Design review of the part built by this model. Coordinates are the model's own, in mm. A direction names the side the tool comes from. Round coordinates to 2 decimals unless told otherwise and drop trailing zeros. Order: outer loops, then holes, each group sorted by start corner. A loop starts at its lowest first (then second) coordinate and runs counter-clockwise, first axis right, second up. Notation, with made-up numbers: (22.5, -34) - (55.5, -34) arc R14 ccw to (55.5, -11) - close; hole circle Ø1 at (78.25, 83). An arc over 180 degrees is marked (long way). Use CSV: the item, a comma, the result in double quotes. Start each with the question number.
from build123d import *

# Parameters (mm, degrees)
BOSS_EXTRUDE3_DEPTH                    = 210
FILLET1_R                              = 2.5
FILLET2_R                              = 12.5
CHAMFER1_SIZE                          = 1
M10_TAPPED_HOLE1_D                     = 8.5
M10_TAPPED_HOLE1_DEPTH                 = 27.5
M10_TAPPED_HOLE1_CSINK_D               = 10.05
M10_TAPPED_HOLE1_CSINK_ANGLE           = 100
M10_TAPPED_HOLE1_TIP                   = 2.553657631
M10_TAPPED_HOLE1_ON_FACE_2_D           = 8.5
M10_TAPPED_HOLE1_ON_FACE_2_DEPTH       = 27.5
M10_TAPPED_HOLE1_ON_FACE_2_CSINK_D     = 10.05
M10_TAPPED_HOLE1_ON_FACE_2_CSINK_ANGLE = 100
M10_TAPPED_HOLE1_ON_FACE_2_TIP         = 2.553657631
CUT_EXTRUDE1_DEPTH                     = 9


with BuildPart() as part:
    # Sketch1 → Boss-Extrude3 (new, symmetric)
    with BuildSketch(Plane(origin=(0, 0, 0), x_dir=(0, 0, -1), z_dir=(1, 0, 0))):
        Polygon((23.094010768, -40), (46.188021535, 0), (23.094010768, 40), (-23.094010768, 40), (-46.188021535, 0), (-23.094010768, -40), align=None)
    extrude(amount=BOSS_EXTRUDE3_DEPTH, both=True)

    # Sketch3 → Revolve1 (revolve)
    with BuildSketch(Plane.XY, mode=Mode.PRIVATE) as revolve1_sk:
        Polygon((-210, 35), (-240, 35), (-240, 32.5), (-265, 32.5), (-265, 0), (-210, 0), align=None)
        Polygon((210, 35), (240, 35), (240, 32.5), (320, 32.5), (320, 30), (420, 30), (420, 0), (210, 0), align=None)
    revolve(revolve1_sk.sketch.rotate(Axis((-265, 0, 0), (1, 0, 0)), 90), axis=Axis((-265, 0, 0), (1, 0, 0)))

    # Fillet1
    fillet1_edges = [part.edges().sort_by_distance(p)[0] for p in [
        (-210, 0, -35),
        (-240, 0, -32.5),
        (210, 0, -35),
        (240, 0, -32.5),
    ]]
    fillet(fillet1_edges, radius=FILLET1_R - 0.0001)  # a hair under: the kernel refuses the full size

    # Fillet2
    fillet2_edges = [part.edges().sort_by_distance(p)[0] for p in [
        (0, -40, 23.094010768),
        (0, 0, 46.188021535),
        (0, 40, 23.094010768),
        (0, 40, -23.094010768),
        (0, 0, -46.188021535),
        (0, -40, -23.094010768),
    ]]
    fillet(fillet2_edges, radius=FILLET2_R)

    # Chamfer1
    chamfer1_edges = [part.edges().sort_by_distance(p)[0] for p in [
        (-265, 0, -32.5),
        (320, 0, -32.5),
        (420, 0, -30),
    ]]
    chamfer(chamfer1_edges, length=CHAMFER1_SIZE)

    # M10 Tapped Hole1
    with Locations(Plane(origin=(-265, 0, 0), x_dir=(0, 0, -1), z_dir=(-1, 0, 0))):
        with Locations((0, 0)):
            CounterSinkHole(M10_TAPPED_HOLE1_D / 2, M10_TAPPED_HOLE1_CSINK_D / 2, depth=M10_TAPPED_HOLE1_DEPTH, counter_sink_angle=M10_TAPPED_HOLE1_CSINK_ANGLE)
            with Locations((0, 0, -(M10_TAPPED_HOLE1_DEPTH + M10_TAPPED_HOLE1_TIP / 2))):  # 118° drill point
                Cone(0, M10_TAPPED_HOLE1_D / 2, M10_TAPPED_HOLE1_TIP, mode=Mode.SUBTRACT)

    # M10 Tapped Hole1 on face 2
    with Locations(Plane(origin=(420, 0, 0), x_dir=(0, 0, 1), z_dir=(1, 0, 0))):
        with Locations((0, 0)):
            CounterSinkHole(M10_TAPPED_HOLE1_ON_FACE_2_D / 2, M10_TAPPED_HOLE1_ON_FACE_2_CSINK_D / 2, depth=M10_TAPPED_HOLE1_ON_FACE_2_DEPTH, counter_sink_angle=M10_TAPPED_HOLE1_ON_FACE_2_CSINK_ANGLE)
            with Locations((0, 0, -(M10_TAPPED_HOLE1_ON_FACE_2_DEPTH + M10_TAPPED_HOLE1_ON_FACE_2_TIP / 2))):  # 118° drill point
                Cone(0, M10_TAPPED_HOLE1_ON_FACE_2_D / 2, M10_TAPPED_HOLE1_ON_FACE_2_TIP, mode=Mode.SUBTRACT)

    # Sketch7 → Cut-Extrude1 (cut)
    with BuildSketch(Plane(origin=(0, 30, 0), x_dir=(1, 0, 0), z_dir=(0, 1, 0))):
        with BuildLine():
            Line((420, -8), (340, -8))
            ThreePointArc((340, -8), (332, 0), (340, 8))
            Line((340, 8), (420, 8))
            ThreePointArc((420, 8), (428, 0), (420, -8))
        make_face()
    extrude(amount=-CUT_EXTRUDE1_DEPTH, mode=Mode.SUBTRACT)


solid = part.part
Q1. Take a section at A-A (x = -128). State the section outline as (y, z) points, plus the area to 3 significant figures.
Q2. Tool access review of faces 5 (the cylindrical face through (370.193, -25.296, 16.128)), 6 (the flat face through (-210, -35.4, -12.9)), 7 (the flat face through (3, 40, 0)): name each direction out of +Z, -Z, +X, -X, +Y, -Y from which nothing blocks a thin tool from reaching the whole face with its end or side.
Q3. For L1, parallel to Y at x = 403.75, z = 0; L2, parallel to Y at x = -244, z = 0; L3, parallel to X at y = 29, z = -12, list the stretches that pass through material, from the lowest coordinate up. Write a range as [from, to].
Q4. Clearance check with flat-ended pins moving along their axes: pin 1 (17.5 mm diameter, centred on x = 386, z = 0.5, fed in from +Y); pin 2 (1 mm diameter, centred on y = -0.5, z = -1.5, fed in from -X); pin 3 (8 mm diameter, centred on y = -26.5, z = 27.5, fed in from -X). State where each tip first meets the part, or that it passes through.
Q5. The part is to be moulded in two halves that separate along Z. For faces 1 (the cylindrical face through (-2.9, -38.4, 22)), 2 (the flat face through (377, 21, 0)), 3 (the flat face through (320, 28, 12)), 4 (the cylindrical face through (226.442, 34.168, -7.587)), say which applies: +Z half, -Z half, draft (parallel to the pull), parting line (faces both ways), or undercut.
Findings below:
1,outline,"(-40, -15.88) arc R12.5 ccw to (-33.75, -26.7) - (-6.25, -42.58) arc R12.5 ccw to (6.25, -42.58) - (33.75, -26.7) arc R12.5 ccw to (40, -15.88) - (40, 15.88) arc R12.5 ccw to (33.75, 26.7) - (6.25, 42.58) arc R12.5 ccw to (-6.25, 42.58) - (-33.75, 26.7) arc R12.5 ccw to (-40, 15.88) - close"
1,area,"5,490 mm^2"
2,face 5,"+X"
2,face 6,"-X"
2,face 7,"+Z, -Z, +X, -X, +Y"
3,L1,"y = [-30, -4.25], [4.25, 21]"
3,L2,"y = [-32.5, -4.25], [4.25, 32.5]"
3,L3,"x = [-265, 320]"
4,pin 1,"stops at y = 28.91"
4,pin 2,"stops at x = -236.2"
4,pin 3,"stops at x = -240.13"
5,face 1,"+Z half"
5,face 2,"undercut"
5,face 3,"draft"
5,face 4,"parting line"
